```python
from build123d import *

# Parameters (mm, degrees)
BOSS_EXTRUDE1_DEPTH      = 6
CUT_EXTRUDE1_DEPTH       = 20
M5_CLEARANCE_HOLE1_D     = 5.3
M5_CLEARANCE_HOLE1_DEPTH = 15
M5_CLEARANCE_HOLE1_TIP   = 1.59228064


with BuildPart() as part:
    # Sketch1 → Boss-Extrude1 (new body)
    with BuildSketch(Plane(origin=(0, 0, 0), x_dir=(0, 0, -1), z_dir=(1, 0, 0))):
        with BuildLine():
            Line((-46.8, 19.5), (-43.038500206, 19.5))
            ThreePointArc((-43.038500206, 19.5), (0, 47.25), (43.038500206, 19.5))
            Line((43.038500206, 19.5), (46.8, 19.5))
            ThreePointArc((46.8, 19.5), (50.7, 0), (46.8, -19.5))
            Line((46.8, -19.5), (43.038500206, -19.5))
            ThreePointArc((43.038500206, -19.5), (0, -47.25), (-43.038500206, -19.5))
            Line((-43.038500206, -19.5), (-46.8, -19.5))
            ThreePointArc((-46.8, -19.5), (-50.7, 0), (-46.8, 19.5))
        make_face()
    extrude(amount=BOSS_EXTRUDE1_DEPTH)

    # Sketch2 → Cut-Extrude1 (cut)
    with BuildSketch(Plane(origin=(6, 0, 0), x_dir=(0, 0, -1), z_dir=(1, 0, 0))):
        with BuildLine():
            ThreePointArc((12, -11.85), (12.707106781, -11.557106781), (13, -10.85))
            Line((13, -10.85), (13, -3.85))
            Line((13, -3.85), (13, 14.15))
            ThreePointArc((13, 14.15), (12.707106781, 14.857106781), (12, 15.15))
            Line((12, 15.15), (-12, 15.15))
            ThreePointArc((-12, 15.15), (-12.707106781, 14.857106781), (-13, 14.15))
            Line((-13, 14.15), (-13, -3.85))
            Line((-13, -3.85), (-13, -10.85))
            ThreePointArc((-13, -10.85), (-12.707106781, -11.557106781), (-12, -11.85))
            Line((-12, -11.85), (12, -11.85))
        make_face()
        with BuildLine():
            Line((-12, -12.85), (12, -12.85))
            ThreePointArc((12, -12.85), (12.707106781, -12.557106781), (13, -11.85))
            Line((13, -11.85), (13, -10.85))
            ThreePointArc((13, -10.85), (12.707106781, -11.557106781), (12, -11.85))
            Line((12, -11.85), (-12, -11.85))
            ThreePointArc((-12, -11.85), (-12.707106781, -11.557106781), (-13, -10.85))
            Line((-13, -10.85), (-13, -11.85))
            ThreePointArc((-13, -11.85), (-12.707106781, -12.557106781), (-12, -12.85))
        make_face()
    extrude(amount=-CUT_EXTRUDE1_DEPTH, mode=Mode.SUBTRACT)

    # M5 Clearance Hole1
    with Locations(Plane.ZY):
        with Locations((-32, 0), (0, 32), (32, 0), (0, -32)):
            Hole(M5_CLEARANCE_HOLE1_D / 2, depth=M5_CLEARANCE_HOLE1_DEPTH)
            with Locations((0, 0, -(M5_CLEARANCE_HOLE1_DEPTH + M5_CLEARANCE_HOLE1_TIP / 2))):  # 118° drill point
                Cone(0, M5_CLEARANCE_HOLE1_D / 2, M5_CLEARANCE_HOLE1_TIP, mode=Mode.SUBTRACT)


solid = part.part
```
Source: CAD feature listing. Evaluate the final solid. Frame: model axes, mm. A direction names the side the tool comes from. Give positions to 0.01 mm unless a question says otherwise; leave off trailing zeros. Write each loop counter-clockwise with the first axis right and the second up, starting at its lowest first coordinate (ties: lowest second). Pieces come first, ordered by that corner, then holes.
1. Section query B-B (y = 0). Return the cut outline in (x, z).
2. First-contact query: pin 1 (3 mm diameter, centred on x = 4, z = -21.5, fed in from +Y); pin 2 (1.8 mm diameter, centred on x = 1.5, z = 3.5, fed in from +Y); pin 3 (3 mm diameter, centred on x = 2.5, y = -26, fed in from +Z). Flat tips, straight axial feed; report the tip coordinate or a pass-through.
3. Section query A-A (z = 0). Return the cut outline in (x, y).
4. Pull-direction query (Z, two-part tool) for faces 1 (the face through (3.04, 34.63, 0.34)), 2 (the face through (2.958, -47.244, -0.758)), 3 (the face through (3, 0.3, -50.7)), 4 (the face through (3, -19.5, -45)); classes: +Z half, -Z half, draft (parallel to the pull), parting line (faces both ways), or undercut.
5. Section query D-D (z = -31). Return the cut outline in (x, y).
6. Section query C-C (x = 3.15). Return the cut outline in (y, z).
7. Material intervals for line 1 along Y through (x, z) = (2.65, 0); line 2 along Y through (x, z) = (2.35, -1.5); line 3 along Y through (x, z) = (3.5, -4.5), sorted ascending.
8. Access query for faces 5 (the face through (3, 19.5, 45)), 6 (the face through (2.958, 47.244, 0.758)), 7 (the face through (3, -12.85, 0)), 8 (the face through (3, -19.5, 45)), 9 (the face through (3, 19.5, -45)). Directions: +Z, -Z, +X, -X, +Y, -Y. A direction counts if a zero-diameter tool reaches every point of the face in a straight line with its end or side. Return the directions, or none.
Output values:
1. outline: (0, -50.7) - (6, -50.7) - (6, -34.65) - (0, -34.65) - close; (0, -29.35) - (6, -29.35) - (6, -13) - (0, -13) - close; (0, 13) - (6, 13) - (6, 29.35) - (0, 29.35) - close; (0, 34.65) - (6, 34.65) - (6, 50.7) - (0, 50.7) - close
2. pin 1: stops at y = 42.81
2. pin 2: stops at y = 47.18
2. pin 3: stops at z = 40.4
3. outline: (0, -47.25) - (6, -47.25) - (6, -34.65) - (0, -34.65) - close; (0, -29.35) - (6, -29.35) - (6, -12.85) - (0, -12.85) - close; (0, 15.15) - (6, 15.15) - (6, 29.35) - (0, 29.35) - close; (0, 34.65) - (6, 34.65) - (6, 47.25) - (0, 47.25) - close
4. face 1: undercut
4. face 2: parting line
4. face 3: -Z half
4. face 4: draft
5. outline: (0, -35.66) - (6, -35.66) - (6, -2.45) - (0, -2.45) - close; (0, 2.45) - (6, 2.45) - (6, 35.66) - (0, 35.66) - close
6. outline: (-19.5, -46.8) arc R50.7 ccw to (19.5, -46.8) - (19.5, -43.04) arc R47.25 ccw to (19.5, 43.04) - (19.5, 46.8) arc R50.7 ccw to (-19.5, 46.8) - (-19.5, 43.04) arc R47.25 ccw to (-19.5, -43.04) - close; hole circle Ø5.3 at (-32, 0); hole (-12.85, -12) arc R1 ccw to (-11.85, -13) - (14.15, -13) arc R1 ccw to (15.15, -12) - (15.15, 12) arc R1 ccw to (14.15, 13) - (-11.85, 13) arc R1 ccw to (-12.85, 12) - close; hole circle Ø5.3 at (0, -32); hole circle Ø5.3 at (0, 32); hole circle Ø5.3 at (32, 0)
7. line 1: y = -47.25 to -34.65, -29.35 to -12.85, 15.15 to 29.35, 34.65 to 47.25
7. line 2: y = -47.23 to -34.18, -29.82 to -12.85, 15.15 to 29.82, 34.18 to 47.23
7. line 3: y = -47.04 to -12.85, 15.15 to 47.04
8. face 5: +Z, +X, -X, +Y
8. face 6: +X, -X, +Y
8. face 7: +X, -X
8. face 8: +Z, +X, -X, -Y
8. face 9: -Z, +X, -X, +Y
